CAD build for the part. Positions are in the model's coordinates, mm. A direction names the side the tool comes from. Coordinates: 2 decimals unless noted, no trailing zeros. Write each loop counter-clockwise with the first axis right and the second up, starting at its lowest first coordinate (ties: lowest second). Pieces come first, ordered by that corner, then holes. Notation, with made-up numbers: (26.25, -36) -> (70.25, -36) arc R6 ccw to (70.25, -32) -> close; hole circle Ø8 at (-25, -20). An arc over 180 degrees is marked (long way). Answer as CSV lines item,"result". Start each with the question number.
```python
from build123d import *

# Parameters (mm, degrees)
SKETCH_1_W          = 88
SKETCH_1_H          = 75
EXTRUDE_1_DEPTH     = 3
SKETCH_2_R          = 1.5
SKETCH_2_R_2        = 1
SKETCH_2_W          = 5.1
SKETCH_2_H          = 40.2
SKETCH_2_R_3        = 2
SKETCH_2_W_2        = 28
SKETCH_2_H_2        = 45
CUT_EXTRUDE_1_DEPTH = 3
FILLET_1_R          = 3


with BuildPart() as part:
    # ｽｹｯﾁ1 → ﾎﾞｽ - 押し出し1 (new body)
    with BuildSketch(Plane(origin=(0, 0, 0), x_dir=(1, 0, 0), z_dir=(0, 1, 0))):
        Rectangle(SKETCH_1_W, SKETCH_1_H)
    extrude(amount=EXTRUDE_1_DEPTH)

    # ｽｹｯﾁ2 → ｶｯﾄ - 押し出し1 (cut)
    with BuildSketch(Plane(origin=(0, 3, 0), x_dir=(1, 0, 0), z_dir=(0, 1, 0))):
        with Locations((-26.5, 32.5)):
            Circle(SKETCH_2_R)
        with Locations((26.5, 32.5)):
            Circle(SKETCH_2_R)
        with Locations((-28.45, -19.5)):
            Circle(SKETCH_2_R_2)
        with Locations((-24.55, -19.5)):
            Circle(SKETCH_2_R_2)
        with Locations((-26.5, 0)):
            Rectangle(SKETCH_2_W, SKETCH_2_H)
        with Locations((-28.45, 19.5)):
            Circle(SKETCH_2_R_2)
        with Locations((-24.55, 19.5)):
            Circle(SKETCH_2_R_2)
        with Locations((26.5, 0)):
            Rectangle(SKETCH_2_W, SKETCH_2_H)
        with Locations((24.55, 19.5)):
            Circle(SKETCH_2_R_2)
        with Locations((28.45, 19.5)):
            Circle(SKETCH_2_R_2)
        with Locations((24.55, -19.5)):
            Circle(SKETCH_2_R_2)
        with Locations((28.45, -19.5)):
            Circle(SKETCH_2_R_2)
        with Locations((-26.5, -32.5)):
            Circle(SKETCH_2_R)
        with Locations((26.5, -32.5)):
            Circle(SKETCH_2_R)
        with Locations((-36.5, -30)):
            Circle(SKETCH_2_R_3)
        with Locations((-36.5, 30)):
            Circle(SKETCH_2_R_3)
        with Locations((36.5, 30)):
            Circle(SKETCH_2_R_3)
        with Locations((36.5, -30)):
            Circle(SKETCH_2_R_3)
        Rectangle(SKETCH_2_W_2, SKETCH_2_H_2)
    extrude(amount=-CUT_EXTRUDE_1_DEPTH, mode=Mode.SUBTRACT)

    # ﾌｨﾚｯﾄ1
    fillet_1_edges = [part.edges().sort_by_distance(p)[0] for p in [
        (-14, 1.5, -22.5),
        (14, 1.5, -22.5),
        (14, 1.5, 22.5),
        (-14, 1.5, 22.5),
    ]]
    fillet(fillet_1_edges, radius=FILLET_1_R)


solid = part.part
```
1. Tool access for faces 1 (the face through (13.14, 1.48, -21.6)), 2 (the face through (44, 1, 1)): list every direction of +Z, -Z, +X, -X, +Y, -Y with a clear straight run to the whole face (end or side of a thin tool).
2. Cut at D-D (x = 26.5). Give the cut face in (y, z), then the cut area to 3 significant figures.
3. Cut at A-A (x = 6.5). Give the cut face in (y, z).
4. Cut at C-C (x = 36.5). Give the cut face in (y, z).
5. Flat gauge pin, fed straight in: P1, Ø1.8, axis at x = 26.5, z = -32.5, coming from the +Y side. Where does the tip first touch, or does it go through?
6. Cut at B-B (z = 5). Give the cut face in (x, y), then the cut area to 3 significant figures.
7. Mould opens along X. For faces 3 (the face through (-20, 3, -1)), 4 (the face through (-44, 1, 1)), 5 (the face through (29.174, 1.521, -20.19)) say: pulls with the +X half, pulls with the -X half, needs draft (parallel to the pull), parting line crosses it, or undercut.
8. Wall check: line 1 (X direction, y = 1.15, z = 18); line 2 (X direction, y = 1.4, z = -30); line 3 (X direction, y = 2, z = -19.5). Give the ranges that are in metal, low to high.
Geometry check:
1,face 1,"+Y, -Y"
1,face 2,"+Z, -Z, +X, +Y, -Y"
2,outline,"(0, -37.5) -> (3, -37.5) -> (3, -34) -> (0, -34) -> close; (0, -31) -> (3, -31) -> (3, -20.1) -> (0, -20.1) -> close; (0, 20.1) -> (3, 20.1) -> (3, 31) -> (0, 31) -> close; (0, 34) -> (3, 34) -> (3, 37.5) -> (0, 37.5) -> close"
2,area,"86.4 mm²"
3,outline,"(0, -37.5) -> (3, -37.5) -> (3, -22.5) -> (0, -22.5) -> close; (0, 22.5) -> (3, 22.5) -> (3, 37.5) -> (0, 37.5) -> close"
4,outline,"(0, -37.5) -> (3, -37.5) -> (3, -32) -> (0, -32) -> close; (0, -28) -> (3, -28) -> (3, 28) -> (0, 28) -> close; (0, 32) -> (3, 32) -> (3, 37.5) -> (0, 37.5) -> close"
5,P1,"through"
6,outline,"(-44, 0) -> (-29.05, 0) -> (-29.05, 3) -> (-44, 3) -> close; (-23.95, 0) -> (-14, 0) -> (-14, 3) -> (-23.95, 3) -> close; (14, 0) -> (23.95, 0) -> (23.95, 3) -> (14, 3) -> close; (29.05, 0) -> (44, 0) -> (44, 3) -> (29.05, 3) -> close"
6,area,"149 mm²"
7,face 3,"needs draft"
7,face 4,"pulls with the -X half"
7,face 5,"undercut"
8,line 1,"-44 to -29.05, -23.95 to -14, 14 to 23.95, 29.05 to 44"
8,line 2,"-44 to -38.5, -34.5 to 34.5, 38.5 to 44"
8,line 3,"-44 to -29.45, -23.55 to -14, 14 to 23.55, 29.45 to 44"
